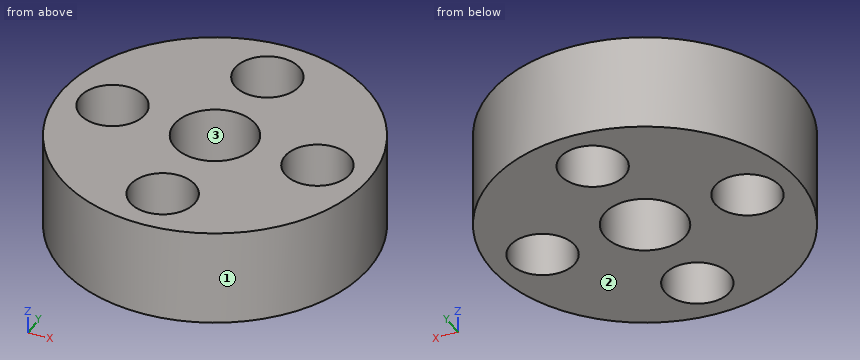
Autodesk Inventor part; units mm, degrees
ref_plane "YZ Plane" through (0, 0, 0) normal (1, 0, 0) x (0, 1, 0)
ref_plane "XZ Plane" through (0, 0, 0) normal (0, 1, 0) x (-1, 0, 0)
ref_plane "XY Plane" through (0, 0, 0) normal (0, 0, 1) x (1, 0, 0)
sketch "Sketch1" plane through (0, 0, 0) normal (0, 0, 1) x (1, 0, 0)
  circle A0 centre (0, 0) radius 9.5
  circle A1 centre (0, 0) radius 2.5
  circle A2 centre (6.35, 0) radius 2
  circle A3 centre (0, 6.35) radius 2
  circle A4 centre (-6.35, 0) radius 2
  circle A5 centre (0, -6.35) radius 2
  dimension "d0" = 19
  dimension "d1" = 5
  dimension "d2" = 4
  dimension "d3" = 6.35
  dimension "d6" = 360
extrude "Extrusion1" add sketch "Sketch1" along normal blind 6
properties part number "HA015" material "ABS Plastic"
Source: CAD feature listing. Evaluate the final solid. Frame: model axes, mm. Face numbers are marked on the shaded views. Coordinates: 2 decimals unless noted, no trailing zeros. Order: outer loops, then holes, each group sorted by start corner. A loop starts at its lowest first (then second) coordinate and runs counter-clockwise, first axis right, second up.
Item 1: Cut plane A-A (x = 0). Return loops of the section in (y, z).
Output values:
outline: (-9.5, 0) - (-8.35, 0) - (-8.35, 6) - (-9.5, 6) - close; (-4.35, 0) - (-2.5, 0) - (-2.5, 6) - (-4.35, 6) - close; (2.5, 0) - (4.35, 0) - (4.35, 6) - (2.5, 6) - close; (8.35, 0) - (9.5, 0) - (9.5, 6) - (8.35, 6) - close
Item 2: Cut plane C-C (x = 6.5). Return loops of the section in (y, z), plus the area to 3 significant figures.
Output values:
outline: (-6.93, 0) - (-1.99, 0) - (-1.99, 6) - (-6.93, 6) - close; (1.99, 0) - (6.93, 0) - (6.93, 6) - (1.99, 6) - close
area: 59.2 mm2
Item 3: Material intervals for line 1 (Y direction, x = 0, z = 1.9); line 2 (Y direction, x = 1.75, z = 5.5); line 3 (X direction, y = -0.75, z = 3.3), sorted ascending.
Output values:
line 1: y = -9.5 to -8.35, -4.35 to -2.5, 2.5 to 4.35, 8.35 to 9.5
line 2: y = -9.34 to -7.32, -5.38 to -1.79, 1.79 to 5.38, 7.32 to 9.34
line 3: x = -9.47 to -8.2, -4.5 to -2.38, 2.38 to 4.5, 8.2 to 9.47
Item 4: Cut plane D-D (z = 4.25). Return loops of the section in (x, y), plus the area to 3 significant figures.
Output values:
outline: circle Ø19 at (0, 0); hole circle Ø4 at (-6.35, 0); hole circle Ø5 at (0, 0); hole circle Ø4 at (0, -6.35); hole circle Ø4 at (0, 6.35); hole circle Ø4 at (6.35, 0)
area: 214 mm2
Item 5: Cut plane B-B (y = -6.35). Return loops of the section in (x, z), plus the area to 3 significant figures.
Output values:
outline: (-7.07, 0) - (-2, 0) - (-2, 6) - (-7.07, 6) - close; (2, 0) - (7.07, 0) - (7.07, 6) - (2, 6) - close
area: 60.8 mm2
Item 6: Pull-direction query (X, two-part tool) for the marked faces 1, 2 and 3; classes: pulls with the +X half, pulls with the -X half, needs draft (parallel to the pull), parting line crosses it, or undercut.
Output values:
face 1: parting line crosses it
face 2: needs draft
face 3: undercut
Item 7: First-contact query: P1, Ø3, axis at x = 2.5, z = 2.5, coming from the +Y side; P2, Ø1, axis at x = -6.5, z = 5.5, coming from the -Y side; P3, Ø1.5, axis at y = -3, z = 5.5, coming from the -X side. Flat tips, straight axial feed; report the tip coordinate or a pass-through.
Output values:
P1: stops at y = 9.45
P2: stops at y = -7.37
P3: stops at x = -9.23
